```python
from build123d import *

# Parameters (mm, degrees)
F1_DEPTH = 19.05
F3_D     = 6.35
F5_D     = 6.35
F5_DEPTH = 12.7
F5_TIP   = 1.9077324654


with BuildPart() as f1:
    # F0 (on Right) → F1 (new body)
    with BuildSketch(Plane.YZ):
        Polygon((0, 38.1), (0, 0), (33.02, 0), (33.02, 38.1), (22.86, 38.1), (22.86, 6.35), (10.16, 6.35), (10.16, 38.1), align=None)
    extrude(amount=F1_DEPTH)

    # F3 (through all)
    with Locations(Plane(origin=(0, 33.02, 0), x_dir=(-1, 0, 0), z_dir=(0, 1, 0))):
        with Locations((-9.5250001177, 25.4)):
            Hole(F3_D / 2)

    # F5
    with Locations(Plane(origin=(0, 0, 0), x_dir=(1, 0, 0), z_dir=(0, 0, -1))):
        with Locations((12.7, -5.08), (12.7, -27.94)):
            Hole(F5_D / 2, depth=F5_DEPTH)
            with Locations((0, 0, -(F5_DEPTH + F5_TIP / 2))):  # 118° drill point
                Cone(0, F5_D / 2, F5_TIP, mode=Mode.SUBTRACT)


solid = f1.part
```
CAD build for the part. Positions are in the model's coordinates, mm. A direction names the side the tool comes from. Give positions to 0.01 mm unless a question says otherwise; leave off trailing zeros. Write each loop counter-clockwise with the first axis right and the second up, starting at its lowest first coordinate (ties: lowest second). Pieces come first, ordered by that corner, then holes. Notation, with made-up numbers: M 43,37.5 L 99,37.5 A9 ccw 99,46.5 Z; hole C -0.5,-16.5 d2. An arc over 180 degrees is marked long. Return JSON: item names as keys, results as strings. Group by question number.
(1) Band-saw the part on A-A (z = 9.5). Give the cut face in (x, y) (3 decimals).
(2) Flat gauge pins, fed straight in: pin 1 Ø4 at (x, z) = (9.525, 25.4) entering from +Y; pin 2 Ø5 at (x, y) = (12.7, 27.94) entering from -Z; pin 3 Ø10 at (x, y) = (9.5, 16.5) entering from +Z. Where does each tip first touch, or does it go through?
(3) Band-saw the part on D-D (y = 19). Give the cut face in (x, z), and give its area (3 significant figures).
(4) Mould opens along Y. For faces 4 (the face through (9, 0, 19)), 5 (the face through (19.05, 24, 19)), 6 (the face through (9, 10.16, 22)) say: pulls with the +Y half, pulls with the -Y half, needs draft (parallel to the pull), parting line crosses it, or undercut.
(5) Band-saw the part on B-B (z = 25.4). Give the cut face in (x, y).
(6) Drill centre lines: L1, parallel to Y at x = 12.7, z = 3.5 (3 decimals); L2, parallel to Y at x = 8.75, z = 9; L3, parallel to X at y = 5, z = 5. Where is each one in solid material? Low to high. Write a range as [from, to].
(7) 3-axis set-ups, long thin cutter, end or side, ignore diameter. For faces 1 (the face through (9, 5, 38.1)), 2 (the face through (9, 17, 6.35)), 3 (the face through (13.39, 31.04, 6.44)): which of +Z, -Z, +X, -X, +Y, -Y reach the whole face in a straight line?
(8) Band-saw the part on C-C (x = 4.5). Give the cut face in (y, z).
Entries:
{
 "1": {"outline": "M 0,0 L 19.05,0 L 19.05,10.16 L 0,10.16 Z; M 0,22.86 L 19.05,22.86 L 19.05,33.02 L 0,33.02 Z; hole C 12.7,5.08 d6.35; hole C 12.7,27.94 d6.35"},
 "2": {"pin 1": "passes through", "pin 2": "stops at z = 13.11", "pin 3": "stops at z = 6.35"},
 "3": {"outline": "M 0,0 L 19.05,0 L 19.05,6.35 L 0,6.35 Z", "area": "121 mm^2"},
 "4": {"face 4": "pulls with the -Y half", "face 5": "needs draft", "face 6": "undercut"},
 "5": {"outline": "M 0,0 L 6.35,0 L 6.35,10.16 L 0,10.16 Z; M 0,22.86 L 6.35,22.86 L 6.35,33.02 L 0,33.02 Z; M 12.7,0 L 19.05,0 L 19.05,10.16 L 12.7,10.16 Z; M 12.7,22.86 L 19.05,22.86 L 19.05,33.02 L 12.7,33.02 Z"},
 "6": {"L1": "y = [0, 1.905], [8.255, 24.765], [31.115, 33.02]", "L2": "y = [0, 10.16], [22.86, 33.02]", "L3": "x = [0, 9.53], [15.87, 19.05]"},
 "7": {"face 1": "+Z, +X, -X, +Y, -Y", "face 2": "+Z, +X, -X", "face 3": "-Z"},
 "8": {"outline": "M 0,0 L 33.02,0 L 33.02,38.1 L 22.86,38.1 L 22.86,6.35 L 10.16,6.35 L 10.16,38.1 L 0,38.1 Z"}
}
